```python
from build123d import *

# Parameters (mm, degrees)
SKETCH1_R           = 3
SKETCH1_R_2         = 4
BOSS_EXTRUDE1_DEPTH = 2.5


with BuildPart() as part:
    # Sketch1 → Boss-Extrude1 (new body)
    with BuildSketch(Plane.XY):
        with BuildLine():
            Line((-1.935375165, 7.76236581), (23.292313718, 14.052335096))
            ThreePointArc((23.292313718, 14.052335096), (26.983786149, 16.783881004), (27.662556702, 21.325640827))
            Line((27.662556702, 21.325640827), (18.953368461, 56.256286973))
            ThreePointArc((18.953368461, 56.256286973), (18.573069496, 59.791447393), (19.164792931, 63.297420849))
            Line((19.164792931, 63.297420849), (34.122984627, 110.913095801))
            ThreePointArc((34.122984627, 110.913095801), (46.372656677, 117.54203466), (53.366264945, 105.496838974))
            Line((53.366264945, 105.496838974), (46.354025639, 63.703511227))
            ThreePointArc((46.354025639, 63.703511227), (46.002134254, 59.983795798), (46.187035414, 56.252050633))
            Line((46.187035414, 56.252050633), (51.60440687, 11.855476374))
            ThreePointArc((51.60440687, 11.855476374), (50.25461519, 6.352759975), (45.598682847, 3.124119492))
            Line((45.598682847, 3.124119492), (1.935375165, -7.76236581))
            ThreePointArc((1.935375165, -7.76236581), (-7.76236581, -1.935375165), (-1.935375165, 7.76236581))
        make_face()
        Circle(SKETCH1_R, mode=Mode.SUBTRACT)
        with Locations((43.663307682, 107.91605793)):
            Circle(SKETCH1_R_2, mode=Mode.SUBTRACT)
        with Locations((31.567212902, 59.401271616)):
            Circle(SKETCH1_R_2, mode=Mode.SUBTRACT)
        with Locations((38.82486977, 88.510143404)):
            Circle(SKETCH1_R, mode=Mode.SUBTRACT)
        with Locations((43.663307682, 10.886485302)):
            Circle(SKETCH1_R, mode=Mode.SUBTRACT)
    extrude(amount=BOSS_EXTRUDE1_DEPTH)


solid = part.part
```
Input: part model. Units: mm. Frame: model coordinates. A direction names the side the tool comes from. Give positions to 0.01 mm unless a question says otherwise; leave off trailing zeros. Order: outer loops, then holes, each group sorted by start corner. A loop starts at its lowest first (then second) coordinate and runs counter-clockwise, first axis right, second up. Notation, with made-up numbers: (37.25, 36.25) - (88.25, 36.25) arc R14 cw to (88.25, 40.25) - close; hole circle Ø9 at (-37.5, -28.5). An arc over 180 degrees is marked (long way). One line per item, written item: value.
1. Draft query along Y for faces 3 (the face through (37, 56, 0)), 4 (the face through (24.073, -2.243, 1.232)), 5 (the face through (48.86, 34.36, 1.23)). Return one class per face: released by +Y, released by -Y, zero draft, split by the parting line, or undercut.
Determined:
face 3: zero draft
face 4: released by -Y
face 5: undercut
2. Pin query (flat end, axial travel): pin 1 Ø5.5 at (x, y) = (0, 0) entering from +Z; pin 2 Ø10.5 at (x, y) = (43.66, 107.92) entering from +Z. Return the tip coordinate at first contact, or that it passes through.
Determined:
pin 1: through
pin 2: z = 2.5
3. Cut plane C-C, the plane y = 0. Output: boundary loops of the cut face in (x, z), and give its area (3 significant figures).
Determined:
outline: (-8, 0) - (-3, 0) - (-3, 2.5) - (-8, 2.5) - close; (3, 0) - (33.07, 0) - (33.07, 2.5) - (3, 2.5) - close
area: 87.7 mm2
4. Reachability of faces 1 (the face through (23.37, 38.55, 1.23)), 2 (the face through (28.619, 62.105, 1.232)) from +Z, -Z, +X, -X, +Y, -Y: full face, straight path, thin tool, end or side. Return the list, or none.
Determined:
face 1: +Z, -Z, -X
face 2: +Z, -Z
5. Cut plane A-A, the plane z = 0.8. Output: boundary loops of the cut face in (x, y).
Determined:
outline: (-1.94, 7.76) arc R8 ccw to (1.94, -7.76) - (45.6, 3.12) arc R8 ccw to (51.6, 11.86) - (46.19, 56.25) arc R26 cw to (46.35, 63.7) - (53.37, 105.5) arc R10 ccw to (34.12, 110.91) - (19.16, 63.3) arc R13 ccw to (18.95, 56.26) - (27.66, 21.33) arc R6 cw to (23.29, 14.05) - close; hole circle Ø6 at (0, 0); hole circle Ø8 at (31.57, 59.4); hole circle Ø6 at (38.82, 88.51); hole circle Ø8 at (43.66, 107.92); hole circle Ø6 at (43.66, 10.89)
6. Line query: probe 1 along X at (y, z) = (56, 0.6); probe 2 along Y at (x, z) = (38, 2.4); probe 3 along Y at (x, z) = (12.5, 0.15). Output: solid intervals per line, ascending.
Determined:
probe 1: 19.02 to 29.46, 33.67 to 46.22
probe 2: 1.23 to 85.63, 91.39 to 116.16
probe 3: -5.13 to 11.36
7. Cut plane D-D, the plane y = 20. Output: boundary loops of the cut face in (x, z).
Determined:
outline: (27.84, 0) - (50.61, 0) - (50.61, 2.5) - (27.84, 2.5) - close
8. Cut plane B-B, the plane x = 0. Output: boundary loops of the cut face in (y, z).
Determined:
outline: (-8, 0) - (-3, 0) - (-3, 2.5) - (-8, 2.5) - close; (3, 0) - (8.24, 0) - (8.24, 2.5) - (3, 2.5) - close
